Geometry: see drawing. Coordinates: mm, zero at the bounding-box minimum. A direction names the side the tool comes from. Give positions to 0.01 mm unless a question says otherwise; leave off trailing zeros. Write each loop counter-clockwise with the first axis right and the second up, starting at its lowest first coordinate (ties: lowest second). Pieces come first, ordered by that corner, then holes.
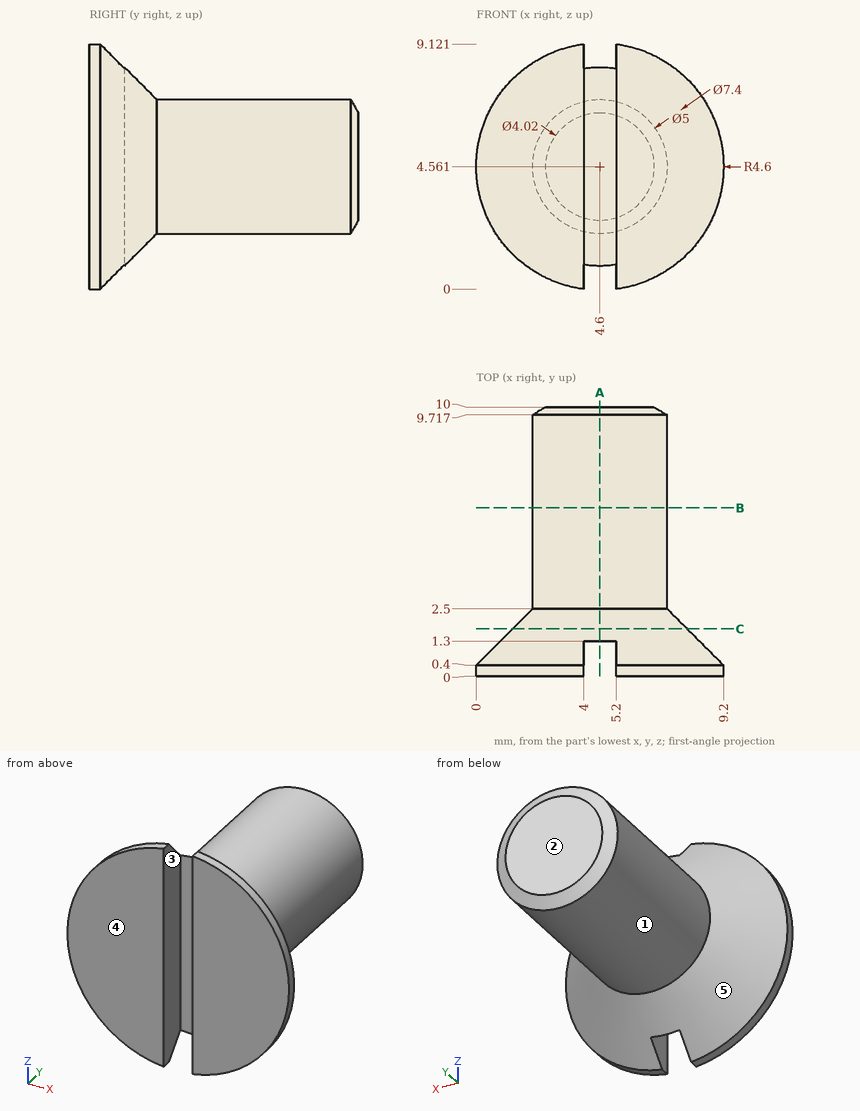
1. Access query for the marked faces 1 and 2. Directions: +Z, -Z, +X, -X, +Y, -Y. A direction counts if a zero-diameter tool reaches every point of the face in a straight line with its end or side. Return the directions, or none.
2. Line query: probe 1 along X at (y, z) = (1, 6.5); probe 2 along X at (y, z) = (3.5, 4.5); probe 3 along X at (y, z) = (1, 6). Output: solid intervals per line, ascending.
3. Section query A-A (x = 4.6). Return loops of the section in (y, z).
4. Section query C-C (y = 1.75). Return loops of the section in (x, z).
5. Section query B-B (y = 6.25). Return loops of the section in (x, z).
6. Pull-direction query (X, two-part tool) for the marked faces 3, 4 and 5; classes: pulls with the +X half, pulls with the -X half, needs draft (parallel to the pull), parting line crosses it, or undercut.
7. Pin query (flat end, axial travel): P1, Ø1.5, axis at y = 5, z = 5.5, coming from the -X side; P2, Ø2, axis at x = 6, z = 1.5, coming from the +Y side (1 decimal); P3, Ø2, axis at y = 8, z = 3, coming from the -X side. Return the tip coordinate at first contact, or that it passes through.
The answers:
1. face 1: +Y
1. face 2: +Z, -Z, +X, -X, +Y
2. probe 1: x = 1.1 to 4, 5.2 to 8.1
2. probe 2: x = 2.1 to 7.1
2. probe 3: x = 0.87 to 4, 5.2 to 8.33
3. outline: (1.3, 0.86) - (2.5, 2.06) - (9.72, 2.06) - (10, 2.55) - (10, 6.57) - (9.72, 7.06) - (2.5, 7.06) - (1.3, 8.26) - close
4. outline: circle Ø6.5 at (4.6, 4.56)
5. outline: circle Ø5 at (4.6, 4.56)
6. face 3: undercut
6. face 4: needs draft
6. face 5: parting line crosses it
7. P1: stops at x = 2.11
7. P2: stops at y = 9.8
7. P3: stops at x = 2.16
